Design review of the part built by this model. Coordinates are the model's own, in mm. A direction names the side the tool comes from. Coordinates: 2 decimals unless noted, no trailing zeros. Loops run counter-clockwise (first coordinate to the right, second up) from the corner with the lowest first, then second, coordinate; pieces in that order, holes last. Notation, with made-up numbers: (84, 82) - (127, 82) arc R20 ccw to (127, 101) - close; hole circle Ø5 at (-27.75, -10.75). An arc over 180 degrees is marked (long way). Use one line per item in the form item = value. Start each with the question number.
(1) Tool access review of faces 1 (the face through (20.683, 9.86, 25.132)), 2 (the face through (15.833, 10, 23)): name each direction out of +Z, -Z, +X, -X, +Y, -Y from which nothing blocks a thin tool from reaching the whole face with its end or side.
(2) Clearance check with flat-ended pins moving along their axes: pin 1 Ø1.5 at (x, y) = (13.5, 17.5) entering from +Z; pin 2 Ø1.5 at (y, z) = (16, 26) entering from +X; pin 3 Ø17.5 at (x, z) = (0, 13.5) entering from +Y; pin 4 Ø10 at (y, z) = (11.5, 24.5) entering from -X. State where each tip first meets the part, or that it passes through.
(3) Add section B-B (y = 8.5). State the section outline as (x, z) points, plus the area to 3 significant figures.
(4) The part is to be moulded in two halves that separate along X. For faces 3 (the face through (0, 40, 0)), 4 (the face through (14.26, 9.86, 7.36)), 5 (the face through (5.78, 29.86, 7.54)), 6 (the face through (-9.281, 9.86, 5.904)), say which applies: pulls with the +X half, pulls with the -X half, needs draft (parallel to the pull), parting line crosses it, or undercut.
(5) Add section D-D (x = 14). State the section outline as (y, z) points.
(6) For L1, parallel to X at y = 38.5, z = 0.5; L2, parallel to Y at x = 19, z = 20; L3, parallel to Z at x = 0, y = 6, list the stretches that pass through material, from the lowest coordinate up.
(7) Add section A-A (z = 7.5). State the section outline as (x, y) points.
(8) Add section C-C (z = -2). State the section outline as (x, y) points.
```python
from build123d import *

# Parameters (mm, degrees)
BOSS_EXTRUDE1_DEPTH = 20
SKETCH4_R           = 9.5
BOSS_EXTRUDE2_DEPTH = 20


with BuildPart() as part:
    # Sketch1 → Boss-Extrude1 (new body)
    with BuildSketch(Plane(origin=(0, 0, 0), x_dir=(1, 0, 0), z_dir=(0, 1, 0))):
        with BuildLine():
            Line((18.424541272, -35.177357689), (23.005994318, -14.800530945))
            ThreePointArc((23.005994318, -14.800530945), (18.132040633, 4.01076546), (0, 11))
            ThreePointArc((0, 11), (-9.097635455, -6.183286273), (10.227869895, -4.048540158))
            ThreePointArc((10.227869895, -4.048540158), (14.304101202, -7.422369294), (15.833057178, -12.488006305))
            Line((15.833057178, -12.488006305), (15.833057178, -33.589930418))
            ThreePointArc((15.833057178, -33.589930418), (16.997270485, -34.598365473), (18.424541272, -35.177357689))
        make_face()
    extrude(amount=BOSS_EXTRUDE1_DEPTH)

    # Sketch4 → Boss-Extrude2 (add)
    with BuildSketch(Plane(origin=(0, 20, 0), x_dir=(1, 0, 0), z_dir=(0, 1, 0))):
        with Locations(Location((0, 0, 0), (0, 0, 90))):
            Circle(SKETCH4_R)
    extrude(amount=BOSS_EXTRUDE2_DEPTH)


solid = part.part
```
Computed values:
q1.face_1 = +Z, +X, +Y, -Y
q1.face_2 = +Z, -X, +Y, -Y
q2.pin_1 = 7.34
q2.pin_2 = 20.66
q2.pin_3 = 40
q2.pin_4 = 15.83
q3.outline = (0, -11) arc R21.26 ccw to (23.01, 14.8) - (18.42, 35.18) arc R4.71 ccw to (15.83, 33.59) - (15.83, 12.49) arc R9.16 cw to (10.23, 4.05) arc R11 ccw (long way) to start
q3.area = 694 mm^2
q4.face_3 = needs draft
q4.face_4 = undercut
q4.face_5 = parting line crosses it
q4.face_6 = undercut
q5.outline = (0, -7.59) - (20, -7.59) - (20, 6.99) - (0, 6.99) - close
q6.L1 = -9.49 to 9.49
q6.L2 = 0 to 20
q6.L3 = -11 to 11
q7.outline = (-8.05, 0) - (8.05, 0) - (8.05, 20) - (5.83, 20) - (5.83, 40) - (-5.83, 40) - (-5.83, 20) - (-8.05, 20) - close; (14.36, 0) - (23.36, 0) - (23.36, 20) - (14.36, 20) - close
q8.outline = (-10.82, 0) - (19.72, 0) - (19.72, 20) - (9.29, 20) - (9.29, 40) - (-9.29, 40) - (-9.29, 20) - (-10.82, 20) - close
